For this review, take the finished solid that the model builds, in its own axes (mm). A direction names the side the tool comes from. Round coordinates to 2 decimals unless told otherwise and drop trailing zeros. Write each loop counter-clockwise with the first axis right and the second up, starting at its lowest first coordinate (ties: lowest second). Pieces come first, ordered by that corner, then holes. Notation, with made-up numbers: (9.5, 18.5) -> (34.5, 18.5) arc R14 cw to (34.5, 34.5) -> close; hole circle Ø2 at (88, -15). An arc over 180 degrees is marked (long way). Answer as CSV lines item,"result". Start each with the question number.
Item 1: Mouldability with a two-part tool opening along X and no side actions: class faces 6 (the flat face through (-35, -27, 3)), 7 (the flat face through (125, 3, 3)), 8 (the flat face through (123, 29.5, 3)) as +X half, -X half, draft (parallel to the pull), parting line (faces both ways), or undercut.
Item 2: Take a section at A-A on x = -4.5. Give the boundary of the cut face in (y, z), then the cut area to 3 significant figures.
Item 3: Machinability: for faces 1 (the flat face through (-120, 26, 3)), 2 (the flat face through (35, -26, 3)), 3 (the flat face through (-2, 0, 6)), 4 (the flat face through (-102, 29.5, 3)), 5 (the flat face through (-85, -26, 3)), which of the approach directions +Z, -Z, +X, -X, +Y, -Y give a long, thin tool a straight path to every point of the face, cutting with its end or side? Answer none if there is none.
Item 4: Wall thickness on probe 1 along Y at (x, z) = (92.5, 5.7); probe 2 along Y at (x, z) = (-41, 2.65): over which ranges is each line inside the solid? List them lowest first. Write a range as from..to.
Item 5: Take a section at B-B on x = 94. Give the boundary of the cut face in (y, z).
Item 6: For pin 1 Ø3 at (x, z) = (41.5, 2) entering from +Y; pin 2 Ø1.8 at (y, z) = (-26.5, 2) entering from +X; pin 3 Ø3 at (x, z) = (102.5, 2.5) entering from -Y, all flat-tipped, find the tip position at first contact; note any pin that passes through.
```python
from build123d import *

# Parameters (mm, degrees)
BOSS_EXTRUDE1_DEPTH = 6
CUT_EXTRUDE1_REACH  = 8
SKETCH2_W           = 20
SKETCH2_H           = 6
SKETCH2_W_2         = 6


with BuildPart() as part:
    # Sketch1 → Boss-Extrude1 (new body)
    with BuildSketch(Plane.XY):
        Polygon((-85, -23.5), (-85, -29.5), (-35, -29.5), (-35, -23.5), (35, -23.5), (35, -29.5), (85, -29.5), (85, -23.5), (125, -23.5), (125, 29.5), (-125, 29.5), (-125, -23.5), align=None)
    extrude(amount=BOSS_EXTRUDE1_DEPTH)

    # Sketch2 → Cut-Extrude1 (cut, up to next)
    with BuildSketch(Plane.XY.offset(6), mode=Mode.PRIVATE) as cut_extrude1_sk1:
        with Locations((-80, 26.5)):
            Rectangle(SKETCH2_W, SKETCH2_H)
    cut_extrude1_tool1 = extrude(cut_extrude1_sk1.sketch, amount=-CUT_EXTRUDE1_REACH, mode=Mode.PRIVATE) & part.part
    add(cut_extrude1_tool1.solids().sort_by_distance((-80, 26.5, 6))[0], mode=Mode.SUBTRACT)
    # Sketch2 → Cut-Extrude1 (cut, up to next)
    with BuildSketch(Plane.XY.offset(6), mode=Mode.PRIVATE) as cut_extrude1_sk2:
        with Locations((-40, 26.5)):
            Rectangle(SKETCH2_W, SKETCH2_H)
    cut_extrude1_tool2 = extrude(cut_extrude1_sk2.sketch, amount=-CUT_EXTRUDE1_REACH, mode=Mode.PRIVATE) & part.part
    add(cut_extrude1_tool2.solids().sort_by_distance((-40, 26.5, 6))[0], mode=Mode.SUBTRACT)
    # Sketch2 → Cut-Extrude1 (cut, up to next)
    with BuildSketch(Plane.XY.offset(6), mode=Mode.PRIVATE) as cut_extrude1_sk3:
        with Locations((0, 26.5)):
            Rectangle(SKETCH2_W, SKETCH2_H)
    cut_extrude1_tool3 = extrude(cut_extrude1_sk3.sketch, amount=-CUT_EXTRUDE1_REACH, mode=Mode.PRIVATE) & part.part
    add(cut_extrude1_tool3.solids().sort_by_distance((0, 26.5, 6))[0], mode=Mode.SUBTRACT)
    # Sketch2 → Cut-Extrude1 (cut, up to next)
    with BuildSketch(Plane.XY.offset(6), mode=Mode.PRIVATE) as cut_extrude1_sk4:
        with Locations((40, 26.5)):
            Rectangle(SKETCH2_W, SKETCH2_H)
    cut_extrude1_tool4 = extrude(cut_extrude1_sk4.sketch, amount=-CUT_EXTRUDE1_REACH, mode=Mode.PRIVATE) & part.part
    add(cut_extrude1_tool4.solids().sort_by_distance((40, 26.5, 6))[0], mode=Mode.SUBTRACT)
    # Sketch2 → Cut-Extrude1 (cut, up to next)
    with BuildSketch(Plane.XY.offset(6), mode=Mode.PRIVATE) as cut_extrude1_sk5:
        with Locations((80, 26.5)):
            Rectangle(SKETCH2_W, SKETCH2_H)
    cut_extrude1_tool5 = extrude(cut_extrude1_sk5.sketch, amount=-CUT_EXTRUDE1_REACH, mode=Mode.PRIVATE) & part.part
    add(cut_extrude1_tool5.solids().sort_by_distance((80, 26.5, 6))[0], mode=Mode.SUBTRACT)
    # Sketch2 → Cut-Extrude1 (cut, up to next)
    with BuildSketch(Plane.XY.offset(6), mode=Mode.PRIVATE) as cut_extrude1_sk6:
        with Locations((-117, 26.5)):
            Rectangle(SKETCH2_W_2, SKETCH2_H)
    cut_extrude1_tool6 = extrude(cut_extrude1_sk6.sketch, amount=-CUT_EXTRUDE1_REACH, mode=Mode.PRIVATE) & part.part
    add(cut_extrude1_tool6.solids().sort_by_distance((-117, 26.5, 6))[0], mode=Mode.SUBTRACT)
    # Sketch2 → Cut-Extrude1 (cut, up to next)
    with BuildSketch(Plane.XY.offset(6), mode=Mode.PRIVATE) as cut_extrude1_sk7:
        with Locations((117, 26.5)):
            Rectangle(SKETCH2_W_2, SKETCH2_H)
    cut_extrude1_tool7 = extrude(cut_extrude1_sk7.sketch, amount=-CUT_EXTRUDE1_REACH, mode=Mode.PRIVATE) & part.part
    add(cut_extrude1_tool7.solids().sort_by_distance((117, 26.5, 6))[0], mode=Mode.SUBTRACT)


solid = part.part
```
Output values:
1,face 6,"undercut"
1,face 7,"+X half"
1,face 8,"draft"
2,outline,"(-23.5, 0) -> (23.5, 0) -> (23.5, 6) -> (-23.5, 6) -> close"
2,area,"282 mm^2"
3,face 1,"+Z, -Z, +Y"
3,face 2,"+Z, -Z, -Y"
3,face 3,"+Z, +X, -X, +Y, -Y"
3,face 4,"+Z, -Z, +X, -X, +Y"
3,face 5,"+Z, -Z, -X, -Y"
4,probe 1,"y = -23.5..29.5"
4,probe 2,"y = -29.5..23.5"
5,outline,"(-23.5, 0) -> (29.5, 0) -> (29.5, 6) -> (-23.5, 6) -> close"
6,pin 1,"stops at y = 23.5"
6,pin 2,"stops at x = 85"
6,pin 3,"stops at y = -23.5"
